Autodesk Inventor part; units mm, degrees
ref_plane "YZ Plane" through (0, 0, 0) normal (1, 0, 0) x (0, 1, 0)
ref_plane "XZ Plane" through (0, 0, 0) normal (0, 1, 0) x (-1, 0, 0)
ref_plane "XY Plane" through (0, 0, 0) normal (0, 0, 1) x (1, 0, 0)
sketch "Sketch1" plane through (0, 0, 0) normal (0, 0, 1) x (1, 0, 0)
  line L0 (-30, -35) -> (-10, -35)
  line L1 (-10, -35) -> (-10, -31)
  line L2 (-10, -31) -> (10, -31)
  line L3 (10, -31) -> (10, -35)
  line L4 (10, -35) -> (30, -35)
  line L5 (30, -35) -> (30, -31)
  line L6 (10, 35) -> (-10, 35)
  line L7 (-30, -31) -> (-30, -35)
  line L8 (-10, 35) -> (-10, 31)
  line L9 (-10, 31) -> (-30, -31)
  line L10 (10, 35) -> (10, 31)
  line L11 (10, 31) -> (30, -31)
  line L12 (-2, 31) -> (2, 31)
  line L13 (2, 31) -> (2, 11)
  line L14 (2, 11) -> (-2, 11)
  line L15 (-2, 11) -> (-2, 31)
  line L16 (2, -11) -> (-2, -11)
  line L17 (-2, -11) -> (-2, -31)
  line L18 (-2, -31) -> (2, -31)
  line L19 (2, -31) -> (2, -11)
  line L20 (0, 31) -> (0, -31) construction
  point P0 (0, 0)
  point P1 (0, 0)
  point P2 (-2, -31)
  point P3 (2, -31)
  dimension "d0" = 4
  dimension "d1" = 20
  dimension "d2" = 20
  dimension "d3" = 20
  dimension "d4" = 20
  dimension "d5" = 4
  dimension "d6" = 4
  dimension "d7" = 62
  dimension "d8" = 20
  dimension "d9" = 20
  dimension "d10" = 4
extrude "Extrusion1" add sketch "Sketch1" along normal blind 4 contours L7 L9 L8 L6 L10 L11 L5 L4 L3 L2 L19 L16 L17 L1 L0
properties part number "LightGate_Plate" material "MDF Medium Density Fiberboard"
Verification items for the finished model (mm, model axes). A direction names the side the tool comes from. Coordinates: 2 decimals unless noted, no trailing zeros. Order: outer loops, then holes, each group sorted by start corner. A loop starts at its lowest first (then second) coordinate and runs counter-clockwise, first axis right, second up. Notation, with made-up numbers: (-5.75, 32.25) -> (34.25, 32.25) arc R23 cw to (34.25, 55.25) -> close; hole circle Ø4 at (-16, 29). An arc over 180 degrees is marked (long way). Put each result on its own line as item: value. Start each with the question number.
1. Cross-section at D-D, the plane y = -30. Record the boundary of the cut face in (x, z).
2. Material ranges on L1, parallel to Y at x = 1, z = 3.15; L2, parallel to Y at x = 6, z = 0.5; L3, parallel to X at y = 21, z = 2.1, recorded low to high. Write a range as [from, to].
3. Cross-section at C-C, the plane x = -25. Record the boundary of the cut face in (y, z), then the cut area to 3 significant figures.
4. Cross-section at B-B, the plane z = 0.65. Record the boundary of the cut face in (x, y).
5. Go/stop test with flat-tipped pins: pin 1 Ø1.2 at (y, z) = (18, 2.5) entering from -X; pin 2 Ø2 at (y, z) = (-25.5, 2.5) entering from +X; pin 3 Ø1.2 at (x, z) = (4, 3) entering from -Y. Record where each tip stops, or that it passes through.
6. Access from +Z, -Z, +X, -X, +Y, -Y to the whole of each face (thin tool, end or side, straight path). Record for faces 1 (the flat face through (0, -11, 2)), 2 (the flat face through (-20, 0, 2)), 3 (the flat face through (0, 11, 2)).
7. Cross-section at A-A, the plane y = 23.5. Record the boundary of the cut face in (x, z).
8. Mould release check, pull along Y, two halves, no side actions. Record for faces 4 (the flat face through (-2, 21, 2)), 5 (the flat face through (6, -31, 2)), 6 (the flat face through (10, -33, 2)): released by +Y, released by -Y, zero draft, split by the parting line, or undercut.
Computed:
1. outline: (-29.68, 0) -> (-2, 0) -> (-2, 4) -> (-29.68, 4) -> close; (2, 0) -> (29.68, 0) -> (29.68, 4) -> (2, 4) -> close
2. L1: [-11, 11], [31, 35]
2. L2: [-31, 35]
2. L3: [-13.23, -2], [2, 13.23]
3. outline: (-35, 0) -> (-15.5, 0) -> (-15.5, 4) -> (-35, 4) -> close
3. area: 78.0 mm2
4. outline: (-30, -35) -> (-10, -35) -> (-10, -31) -> (-2, -31) -> (-2, -11) -> (2, -11) -> (2, -31) -> (10, -31) -> (10, -35) -> (30, -35) -> (30, -31) -> (10, 31) -> (10, 35) -> (-10, 35) -> (-10, 31) -> (-30, -31) -> close; hole (-2, 11) -> (2, 11) -> (2, 31) -> (-2, 31) -> close
5. pin 1: x = -14.39
5. pin 2: x = 28.55
5. pin 3: y = -31
6. face 1: +Z, -Z, -Y
6. face 2: +Z, -Z, -X, +Y
6. face 3: +Z, -Z
7. outline: (-12.42, 0) -> (-2, 0) -> (-2, 4) -> (-12.42, 4) -> close; (2, 0) -> (12.42, 0) -> (12.42, 4) -> (2, 4) -> close
8. face 4: undercut
8. face 5: released by -Y
8. face 6: zero draft
